Can you work these out from the drawing? Everything is in mm from the part's minimum corner. Give positions to 0.01 mm unless a question says otherwise; leave off trailing zeros. Order: outer loops, then holes, each group sorted by start corner. A loop starts at its lowest first (then second) coordinate and runs counter-clockwise, first axis right, second up. Notation, with made-up numbers: M 57.25,59 L 80.25,59 A9 ccw 80.25,68 Z; hole C 59.5,70 d10. An arc over 180 degrees is marked long. Answer as a JSON object with one key per item and string values.
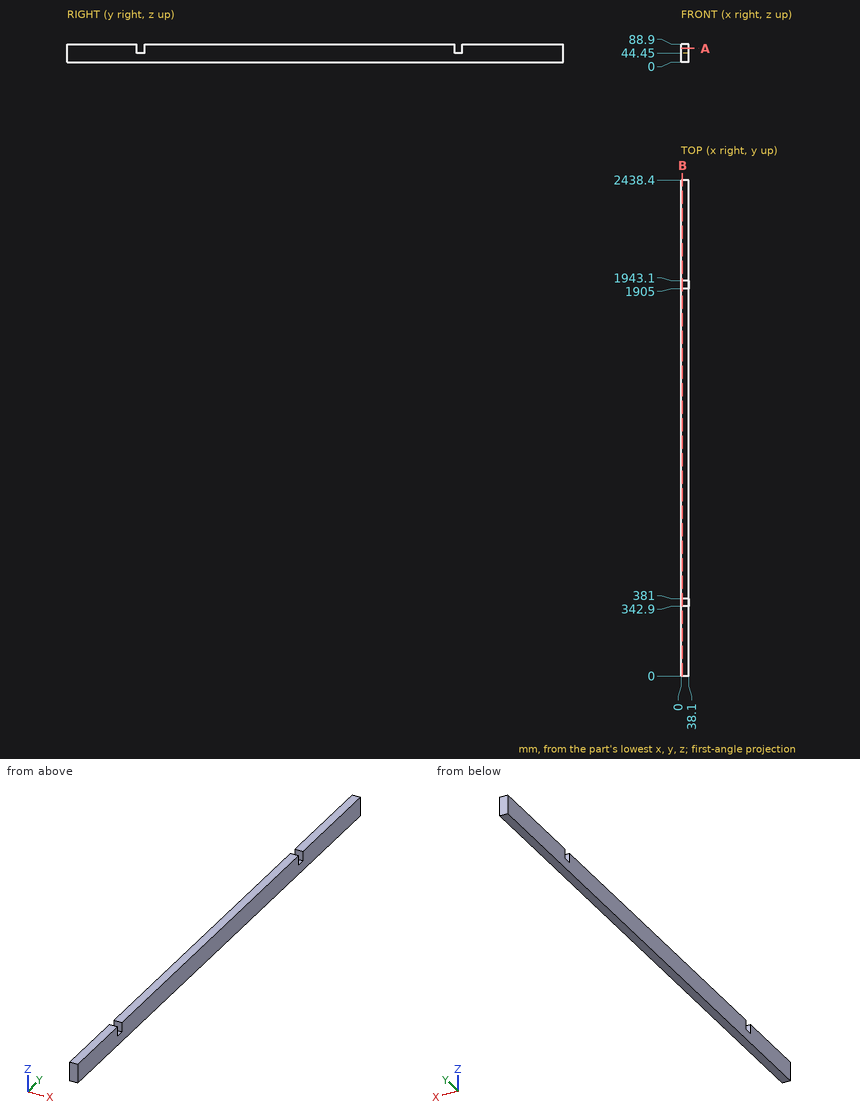
1) I want a section at B-B on x = 6. Write out the boundary of the cut face in (y, z).
Results found:
{"outline": "M 0,0 L 2438.4,0 L 2438.4,88.9 L 1943.1,88.9 L 1943.1,44.45 L 1905,44.45 L 1905,88.9 L 381,88.9 L 381,44.45 L 342.9,44.45 L 342.9,88.9 L 0,88.9 Z"}
2) I need wall thicknesses on L1, parallel to Y at x = 9, z = 57. Which ranges of the line are inside material? Lowest first, please.
Results found:
{"L1": "y = 0 to 342.9, 381 to 1905, 1943.1 to 2438.4"}
3) I want a section at A-A on z = 67. Write out the boundary of the cut face in (x, y).
Results found:
{"outline": "M 0,0 L 38.1,0 L 38.1,342.9 L 0,342.9 Z; M 0,381 L 38.1,381 L 38.1,1905 L 0,1905 Z; M 0,1943.1 L 38.1,1943.1 L 38.1,2438.4 L 0,2438.4 Z"}
4) I'm going to push flat-ended pins straight in: pin 1 Ø12 at (x, z) = (30, 67) entering from -Y; pin 2 Ø11.5 at (x, y) = (15.5, 367) entering from +Z. Where does each tip first touch, or does it pass through?
Results found:
{"pin 1": "stops at y = 0", "pin 2": "stops at z = 44.45"}
